Could you check a few things on this model? Use its own coordinates, in mm. Round coordinates to 2 decimals unless told otherwise and drop trailing zeros. Write each loop counter-clockwise with the first axis right and the second up, starting at its lowest first coordinate (ties: lowest second). Pieces come first, ordered by that corner, then holes. Notation, with made-up numbers: (46, 23.25) - (88, 23.25) arc R20 cw to (88, 27.25) - close; hole circle Ø3 at (59.5, 10.25). An arc over 180 degrees is marked (long way). Put each result on its own line as item: value.
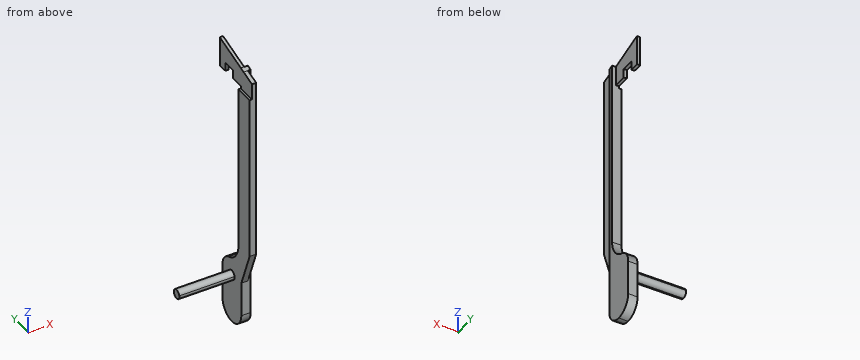
from build123d import *

# Parameters (mm, degrees)
SKETCH1_W           = 45.72
SKETCH1_H           = 1.27
BOSS_EXTRUDE2_DEPTH = 2.54
SKETCH1_5_W         = 45.72
SKETCH1_5_H         = 3.81
BOSS_EXTRUDE3_DEPTH = 1.778
BOSS_EXTRUDE4_START = 1.524
BOSS_EXTRUDE4_DEPTH = 1.27
SKETCH2_W           = 0.634140794
SKETCH2_H           = 8.731528753
CUT_EXTRUDE1_DEPTH  = 75.912777682
BOSS_EXTRUDE5_DEPTH = 14.986


with BuildPart() as part:
    # Sketch1 → Boss-Extrude2 (new body)
    with BuildSketch(Plane(origin=(0, 0, 0), x_dir=(0, 0, -1), z_dir=(1, 0, 0))):
        with BuildLine():
            ThreePointArc((4.318, 0), (3.053287081, 3.053287081), (0, 4.318))
            Line((0, 4.318), (0, -4.318))
            ThreePointArc((0, -4.318), (3.053287081, -3.053287081), (4.318, 0))
        make_face()
        with BuildLine():
            Line((0, -4.318), (0, 4.318))
            ThreePointArc((0, 4.318), (-4.318, 0), (0, -4.318))
        make_face()
        with BuildLine():
            ThreePointArc((0, -4.318), (-4.318, 0), (0, 4.318))
            Line((0, 4.318), (-9.398, 4.318))
            Line((-9.398, 4.318), (-9.398, 1.244340789))
            ThreePointArc((-9.398, 1.244340789), (-8.340781474, 0.98373777), (-7.874, 0))
            ThreePointArc((-7.874, 0), (-8.340781474, -0.98373777), (-9.398, -1.244340789))
            Line((-9.398, -1.244340789), (-9.398, -4.318))
            Line((-9.398, -4.318), (0, -4.318))
        make_face()
        with BuildLine():
            Line((-9.398, 1.244340789), (-9.398, 4.318))
            ThreePointArc((-9.398, 4.318), (-11.932525974, 3.495897895), (-13.501957395, 1.342630889))
            ThreePointArc((-13.501957395, 1.342630889), (-15.817903355, -1.834857441), (-19.558, -3.048))
            Line((-19.558, -3.048), (-19.558, -4.318))
            Line((-19.558, -4.318), (-9.398, -4.318))
            Line((-9.398, -4.318), (-9.398, -1.244340789))
            ThreePointArc((-9.398, -1.244340789), (-10.414, 0), (-9.398, 1.244340789))
        make_face()
        with Locations((-42.418, -3.683)):
            Rectangle(SKETCH1_W, SKETCH1_H)
        Polygon((-70.187321023, -4.318), (-65.278, -4.318), (-65.278, -3.048), (-70.56158602, -3.048), align=None)
        with BuildLine():
            ThreePointArc((-7.874, 0), (-8.340781474, 0.98373777), (-9.398, 1.244340789))
            Line((-9.398, 1.244340789), (-9.398, -1.244340789))
            ThreePointArc((-9.398, -1.244340789), (-8.340781474, -0.98373777), (-7.874, 0))
        make_face()
        with BuildLine():
            Line((-9.398, -1.244340789), (-9.398, 1.244340789))
            ThreePointArc((-9.398, 1.244340789), (-10.414, 0), (-9.398, -1.244340789))
        make_face()
    extrude(amount=BOSS_EXTRUDE2_DEPTH)

    # Sketch1_5 → Boss-Extrude3 (add)
    with BuildSketch(Plane(origin=(0, 0, 0), x_dir=(0, 0, -1), z_dir=(1, 0, 0))):
        Polygon((-19.558, -8.128), (-9.398, -4.318), (-19.558, -4.318), align=None)
        with Locations((-42.418, -6.223)):
            Rectangle(SKETCH1_5_W, SKETCH1_5_H)
        Polygon((-69.06452603, -8.128), (-65.278, -8.128), (-65.278, -4.318), (-70.187321023, -4.318), align=None)
    extrude(amount=BOSS_EXTRUDE3_DEPTH)

    # Sketch1_7 → Boss-Extrude4 (add)
    with BuildSketch(Plane(origin=(0, 0, 0), x_dir=(0, 0, -1), z_dir=(1, 0, 0)).offset(BOSS_EXTRUDE4_START)):
        Polygon((-70.56158602, -3.048), (-65.278, -3.048), (-65.278, 0.508), (-67.708502007, 0.508), (-67.708502007, 4.064), (-65.278, 4.064), (-65.278, 6.604), (-73.406, 6.604), align=None)
    extrude(amount=-BOSS_EXTRUDE4_DEPTH)

    # Sketch2 → Cut-Extrude1 (cut, through all)
    with BuildSketch(Plane(origin=(0, 6.604, 0), x_dir=(1, 0, 0), z_dir=(0, 1, 0))):
        with Locations((0.317070397, -69.040235623)):
            Rectangle(SKETCH2_W, SKETCH2_H)
    extrude(amount=-CUT_EXTRUDE1_DEPTH, mode=Mode.SUBTRACT)

    # Sketch1_8 → Boss-Extrude5 (add)
    with BuildSketch(Plane(origin=(0, 0, 0), x_dir=(0, 0, -1), z_dir=(1, 0, 0))):
        with BuildLine():
            ThreePointArc((-7.874, 0), (-8.340781474, 0.98373777), (-9.398, 1.244340789))
            Line((-9.398, 1.244340789), (-9.398, -1.244340789))
            ThreePointArc((-9.398, -1.244340789), (-8.340781474, -0.98373777), (-7.874, 0))
        make_face()
        with BuildLine():
            Line((-9.398, -1.244340789), (-9.398, 1.244340789))
            ThreePointArc((-9.398, 1.244340789), (-10.414, 0), (-9.398, -1.244340789))
        make_face()
    extrude(amount=-BOSS_EXTRUDE5_DEPTH)


solid = part.part
(1) I'm going to push flat-ended pins straight in: pin 1 (10 mm diameter, centred on x = -6.5, z = 48, fed in from -Y); pin 2 (2.5 mm diameter, centred on y = -3, z = 68.5, fed in from -X); pin 3 (10 mm diameter, centred on x = -0.5, z = 53, fed in from +Y); pin 4 (3 mm diameter, centred on y = -6.5, z = 31.5, fed in from +X). Where does each tip first touch, or does it pass through?
Values found:
pin 1: passes through
pin 2: stops at x = 0.63
pin 3: stops at y = -3.05
pin 4: stops at x = 1.78
(2) Imagine slicing it at A-A, the plane x = -13.5. List the corners of the cut face in (y, z) for me.
Values found:
outline: circle Ø2.54 at (0, 9.14)
(3) Imagine slicing it at B-B, the plane z = 5. List the corners of the cut face in (x, y) for me, then the cut area to 3 significant figures.
Values found:
outline: (0, -4.32) - (2.54, -4.32) - (2.54, 4.32) - (0, 4.32) - close
area: 21.9 mm^2
(4) Please list where these lines run through material, in increasing order: probe 1 along X at (y, z) = (-4, 60.5); probe 2 along X at (y, z) = (-7.25, 59); probe 3 along Z at (x, y) = (-7.75, -0.25). Write a range as from..to.
Values found:
probe 1: x = 0..2.54
probe 2: x = 0..1.78
probe 3: z = 7.9..10.39
(5) Imagine slicing it at D-D, the plane z = 42.5. List the corners of the cut face in (x, y) for me, then the cut area to 4 significant figures.
Values found:
outline: (0, -8.13) - (1.78, -8.13) - (1.78, -4.32) - (2.54, -4.32) - (2.54, -3.05) - (0, -3.05) - close
area: 10.00 mm^2
(6) Imagine slicing it at C-C, the plane y = -5.5. List the corners of the cut face in (x, z) for me, then the cut area to 3 significant figures.
Values found:
outline: (0, 12.55) - (1.78, 12.55) - (1.78, 69.84) - (0.63, 69.84) - (0.63, 64.67) - (0, 64.67) - close
area: 98.6 mm^2
